The model under review builds one solid part; all positions refer to its coordinate system, in mm. A direction names the side the tool comes from. Give positions to 0.01 mm unless a question says otherwise; leave off trailing zeros. Order: outer loops, then holes, each group sorted by start corner. A loop starts at its lowest first (then second) coordinate and runs counter-clockwise, first axis right, second up. Notation, with made-up numbers: (43.25, 17) - (87.25, 17) arc R14 ccw to (87.25, 32) - close; hole circle Ø2 at (19, 38.25). An arc over 180 degrees is marked (long way). Put each result on its own line as item: value.
Autodesk Inventor part; units mm, degrees
ref_plane "YZ Plane" through (0, 0, 0) normal (1, 0, 0) x (0, 1, 0)
ref_plane "XZ Plane" through (0, 0, 0) normal (0, 1, 0) x (-1, 0, 0)
ref_plane "XY Plane" through (0, 0, 0) normal (0, 0, 1) x (1, 0, 0)
ref_plane "Arbeitsebene1" through (0, 0, 0) normal (0, 0, 1) x (1, 0, 0)
sketch "Skizze1" plane through (0, 0, 0) normal (0, 0, 1) x (1, 0, 0)
  line L0 (31.9586, -24.4) -> (31.9586, -21.8494)
  line L1 (31.9586, -24.4) -> (35.5793, -24.4)
  arc A0 (35.5793, -24.4) -> (36.5793, -23.4) centre (35.5793, -23.4) ccw
  line L2 (36.5793, -23.4) -> (36.5793, 14.6)
  arc A1 (36.5793, 14.6) -> (35.5793, 15.6) centre (35.5793, 14.6) ccw
  line L3 (35.5793, 15.6) -> (31.5586, 15.6)
  line L4 (31.5586, 15.6) -> (31.5586, -0.3724)
  arc A2 (32.766, -2.6793) -> (31.5586, -0.3724) centre (29.9586, -2.6793) ccw
  line L5 (32.766, -2.6793) -> (32.766, -19.8793)
  arc A3 (31.9586, -21.8494) -> (32.766, -19.8793) centre (29.9586, -19.8793) ccw
  line L6 (20.9586, -22.6867) -> (20.9586, -24.4)
  line L7 (20.9586, -22.6867) -> (16.1586, -22.6867)
  arc A4 (13.3512, -19.8793) -> (16.1586, -22.6867) centre (16.1586, -19.8793) ccw
  line L8 (13.3512, -19.8793) -> (13.3512, -2.6793)
  arc A5 (14.5586, -0.3724) -> (13.3512, -2.6793) centre (16.1586, -2.6793) ccw
  line L9 (14.5586, -0.3724) -> (14.5586, 15.6)
  line L10 (14.5586, 15.6) -> (10.5793, 15.6)
  arc A6 (10.5793, 15.6) -> (9.5793, 14.6) centre (10.5793, 14.6) ccw
  line L11 (9.5793, 14.6) -> (9.5793, -23.4)
  arc A7 (9.5793, -23.4) -> (10.5793, -24.4) centre (10.5793, -23.4) ccw
  line L12 (10.5793, -24.4) -> (20.9586, -24.4)
  circle A8 centre (12.0668, 4.4966) radius 1.4
  line L13 (31.5586, 15.6) -> (14.5586, 15.6)
  line L14 (31.9586, -24.4) -> (20.9586, -24.4)
  line L15 (10.5793, 15.6) -> (9.5793, 15.6)
  line L16 (9.5793, 15.6) -> (9.5793, 14.6)
  line L17 (35.5793, 15.6) -> (36.5793, 15.6)
  line L18 (36.5793, 15.6) -> (36.5793, 14.6)
  line L19 (9.5793, -23.4) -> (9.5793, -24.4)
  line L20 (9.5793, -24.4) -> (10.5793, -24.4)
  line L21 (35.5793, -24.4) -> (36.5793, -24.4)
  line L22 (36.5793, -24.4) -> (36.5793, -23.4)
extrude "Extrusion1" add sketch "Skizze1" along normal blind 2 contours L14 L6 L7 A4 L8 A5 L9 L13 L4 A2 L5 A3 L0 | L0 A3 L5 A2 L4 L3 A1 L2 A0 L1 | A0 L22 L21 | L12 A7 L11 A6 L10 L9 A5 L8 A4 L7 L6 | L20 L19 A7 | A1 L17 L18 | L16 L15 A6 | A8
ref_plane "Arbeitsebene2" through (0, 0, 0) normal (0, 0, 1) x (1, 0, 0)
sketch "Skizze2" plane through (0, 0, 2) normal (0, 0, 1) x (1, 0, 0)
  arc A0 (35.5793, -24.4) -> (36.5793, -23.4) centre (35.5793, -23.4) ccw
  line L0 (36.5793, -23.4) -> (36.5793, 14.6)
  arc A1 (36.5793, 14.6) -> (35.5793, 15.6) centre (35.5793, 14.6) ccw
  line L1 (35.5793, 15.6) -> (10.5793, 15.6)
  arc A2 (10.5793, 15.6) -> (9.5793, 14.6) centre (10.5793, 14.6) ccw
  line L2 (9.5793, 14.6) -> (9.5793, -23.4)
  arc A3 (9.5793, -23.4) -> (10.5793, -24.4) centre (10.5793, -23.4) ccw
  line L3 (10.5793, -24.4) -> (35.5793, -24.4)
  line L4 (34.0793, 13.1) -> (34.0793, -21.9)
  line L5 (34.0793, -21.9) -> (12.0793, -21.9)
  line L6 (12.0793, -21.9) -> (12.0793, 13.1)
  line L7 (12.0793, 13.1) -> (34.0793, 13.1)
  point P0 (8.0712, 15)
  point P1 (8.0712, -15)
  point P2 (38.0712, 15)
  point P3 (38.0712, -15)
  dimension "d21" = 2.5
hole "Bohrung1" at (34.0793, 13.1, 2) at (34.0793, -21.9, 2) at (12.0793, -21.9, 2) at (12.0793, 13.1, 2) direction (0, 0, -1) diameter 3.2 end through all
sketch "Skizze4" plane through (0, 0, 0) normal (0, 0, -1) x (-1, 0, 0)
  circle A0 centre (-34.0793, 13.1) radius 1.4
  circle A1 centre (-34.0793, -21.9) radius 1.4
  line L0 (-31.9586, -24.4) -> (-31.9586, -21.8494)
  line L1 (-31.9586, -24.4) -> (-35.5793, -24.4)
  arc A2 (-36.5793, -23.4) -> (-35.5793, -24.4) centre (-35.5793, -23.4) ccw
  line L2 (-36.5793, -23.4) -> (-36.5793, 14.6)
  arc A3 (-35.5793, 15.6) -> (-36.5793, 14.6) centre (-35.5793, 14.6) ccw
  line L3 (-35.5793, 15.6) -> (-31.5586, 15.6)
  line L4 (-31.5586, 15.6) -> (-31.5586, -0.3724)
  arc A4 (-31.5586, -0.3724) -> (-32.766, -2.6793) centre (-29.9586, -2.6793) ccw
  line L5 (-32.766, -2.6793) -> (-32.766, -19.8793)
  arc A5 (-32.766, -19.8793) -> (-31.9586, -21.8494) centre (-29.9586, -19.8793) ccw
  circle A6 centre (-12.0793, -21.9) radius 1.4
  circle A7 centre (-12.0793, 13.1) radius 1.4
  line L6 (-20.9586, -22.6867) -> (-20.9586, -24.4)
  line L7 (-20.9586, -22.6867) -> (-16.1586, -22.6867)
  arc A8 (-16.1586, -22.6867) -> (-13.3512, -19.8793) centre (-16.1586, -19.8793) ccw
  line L8 (-13.3512, -19.8793) -> (-13.3512, -2.6793)
  arc A9 (-13.3512, -2.6793) -> (-14.5586, -0.3724) centre (-16.1586, -2.6793) ccw
  line L9 (-14.5586, -0.3724) -> (-14.5586, 15.6)
  line L10 (-14.5586, 15.6) -> (-10.5793, 15.6)
  arc A10 (-9.5793, 14.6) -> (-10.5793, 15.6) centre (-10.5793, 14.6) ccw
  line L11 (-9.5793, 14.6) -> (-9.5793, -23.4)
  arc A11 (-10.5793, -24.4) -> (-9.5793, -23.4) centre (-10.5793, -23.4) ccw
  line L12 (-10.5793, -24.4) -> (-20.9586, -24.4)
  circle A12 centre (-12.0668, 4.4966) radius 1.4
  line L13 (-31.0586, -0.651) -> (-31.0586, 16.1)
  line L14 (-31.0586, 16.1) -> (-35.5793, 16.1)
  arc A13 (-35.5793, 16.1) -> (-37.0793, 14.6) centre (-35.5793, 14.6) ccw
  line L15 (-37.0793, 14.6) -> (-37.0793, -23.4)
  arc A14 (-37.0793, -23.4) -> (-35.5793, -24.9) centre (-35.5793, -23.4) ccw
  line L16 (-35.5793, -24.9) -> (-31.4586, -24.9)
  line L17 (-31.4586, -24.9) -> (-31.4586, -21.6326)
  arc A15 (-32.266, -19.8793) -> (-31.4586, -21.6326) centre (-29.9586, -19.8793) ccw
  line L18 (-32.266, -19.8793) -> (-32.266, -2.6793)
  arc A16 (-31.0586, -0.651) -> (-32.266, -2.6793) centre (-29.9586, -2.6793) ccw
  line L19 (-15.0586, 16.1) -> (-15.0586, -0.651)
  arc A17 (-13.8512, -2.6793) -> (-15.0586, -0.651) centre (-16.1586, -2.6793) ccw
  line L20 (-13.8512, -2.6793) -> (-13.8512, -19.8793)
  arc A18 (-16.1586, -22.1867) -> (-13.8512, -19.8793) centre (-16.1586, -19.8793) ccw
  line L21 (-16.1586, -22.1867) -> (-21.4586, -22.1867)
  line L22 (-21.4586, -24.4607) -> (-21.4586, -24.9)
  line L23 (-21.4586, -24.9) -> (-10.5793, -24.9)
  arc A19 (-10.5793, -24.9) -> (-9.0793, -23.4) centre (-10.5793, -23.4) ccw
  line L24 (-9.0793, -23.4) -> (-9.0793, 14.6)
  arc A20 (-9.0793, 14.6) -> (-10.5793, 16.1) centre (-10.5793, 14.6) ccw
  line L25 (-10.5793, 16.1) -> (-15.0586, 16.1)
  line L26 (-31.0586, 15.6607) -> (-15.0586, 15.6607)
  line L27 (-31.4586, -24.4607) -> (-21.4586, -24.4607)
  line L28 (-15.0586, -0.651) -> (-31.0586, -0.651)
  line L29 (-20.9586, -22.6867) -> (-20.9586, -22.1867)
  line L30 (-20.9586, -22.1867) -> (-31.9586, -22.1867)
  point P0 (0, 0)
  point P1 (-31.4586, -22.1867)
  dimension "d22" = 0.5
  dimension "d23" = 0.5
extrude "Extrusion2" add sketch "Skizze4" along normal blind 3 contours L17 A15 L18 A16 L28 A17 L20 A18 L21 L30
fillet "Rundung2" radius 4 4 edges at (9.5793, 15.6, 1) (36.5793, 15.6, 1) (9.5793, -24.4, 1) (36.5793, -24.4, 1)
sketch "Skizze5" plane through (0, 0, 0) normal (0, 0, -1) x (-1, 0, 0)
  circle A0 centre (-23.0793, -4.4) radius 4.25
  circle A1 centre (-12.0668, 4.4966) radius 1.4
  circle A2 centre (-34.0668, 4.4966) radius 1.4
  circle A3 centre (-12.0793, 13.1) radius 1.4
  circle A4 centre (-34.0793, -21.9) radius 1.4
  circle A5 centre (-34.0793, 13.1) radius 1.4
  circle A6 centre (-12.0793, -21.9) radius 1.4
  arc A7 (-29.0793, 13.6) -> (-31.0793, 15.6) centre (-31.0793, 13.6) ccw
  line L0 (-32.5793, 15.6) -> (-31.0793, 15.6)
  arc A8 (-32.5793, 15.6) -> (-36.5793, 11.6) centre (-32.5793, 11.6) ccw
  line L1 (-36.5793, -20.4) -> (-36.5793, 11.6)
  arc A9 (-36.5793, -20.4) -> (-32.5793, -24.4) centre (-32.5793, -20.4) ccw
  line L2 (-13.5793, -24.4) -> (-32.5793, -24.4)
  arc A10 (-13.5793, -24.4) -> (-9.5793, -20.4) centre (-13.5793, -20.4) ccw
  line L3 (-9.5793, 11.6) -> (-9.5793, -20.4)
  arc A11 (-9.5793, 11.6) -> (-13.5793, 15.6) centre (-13.5793, 11.6) ccw
  line L4 (-15.0793, 15.6) -> (-13.5793, 15.6)
  arc A12 (-15.0793, 15.6) -> (-17.0793, 13.6) centre (-15.0793, 13.6) ccw
  line L5 (-17.0793, 13.6) -> (-17.0793, 5.6)
  arc A13 (-19.0793, 3.6) -> (-17.0793, 5.6) centre (-19.0793, 5.6) ccw
  line L6 (-19.0793, 3.6) -> (-27.0793, 3.6)
  arc A14 (-29.0793, 5.6) -> (-27.0793, 3.6) centre (-27.0793, 5.6) ccw
  line L7 (-29.0793, 5.6) -> (-29.0793, 13.6)
  line L8 (-32.5793, 15.6) -> (-13.5793, 15.6)
  point P0 (0, 0)
extrude "Extrusion3" cut sketch "Skizze5" against normal blind 10 contours A7 L8 A12 L5 A13 L6 A14 L7
properties part number "00_ESP32_XIAO_Adapter_lid"
(1) Clearance check with flat-ended pins moving along their axes: pin 1 Ø2.5 at (x, z) = (23, -1) entering from +Y; pin 2 Ø1 at (x, z) = (31.5, -1.5) entering from -Y; pin 3 Ø0.9 at (y, z) = (-11.5, -1.5) entering from -X; pin 4 Ø5 at (x, y) = (34.08, 13.1) entering from +Z. State where each tip first meets the part, or that it passes through.
The answers:
pin 1: y = 3.6
pin 2: y = -22.19
pin 3: x = 13.85
pin 4: z = 2
(2) Take a section at B-B, the plane z = -2.3. Write out the cut boundary in (x, y), then the cut area to 3 significant figures.
The answers:
outline: (13.85, -19.88) arc R2.31 ccw to (16.16, -22.19) - (31.46, -22.19) - (31.46, -21.63) arc R2.31 ccw to (32.27, -19.88) - (32.27, -2.68) arc R2.31 ccw to (31.06, -0.65) - (15.06, -0.65) arc R2.31 ccw to (13.85, -2.68) - close
area: 393 mm^2
(3) Wall thickness on L1, parallel to X at y = 12, z = 1.05; L2, parallel to X at y = 13.1, z = 1.2; L3, parallel to Y at x = 11.5, z = 0.7: over which ranges is each line inside the solid? List them lowest first.
The answers:
L1: 9.6 to 10.92, 13.24 to 17.08, 29.08 to 32.92, 35.24 to 36.56
L2: 9.87 to 10.48, 13.68 to 17.08, 29.08 to 32.48, 35.68 to 36.29
L3: -23.82 to -23.39, -20.41 to 11.61, 14.59 to 15.02
(4) Take a section at C-C, the plane x = 22.25. Write out the cut boundary in (y, z).
The answers:
outline: (-24.4, 0) - (-22.19, 0) - (-22.19, -3) - (-0.65, -3) - (-0.65, 0) - (3.6, 0) - (3.6, 2) - (-24.4, 2) - close
(5) The part is to be moulded in two halves that separate along Y. For faces 1 (the cylindrical face through (11.599, 11.574, 0.986)), 2 (the flat face through (24, -22.187, -1)), 3 (the cylindrical face through (33.599, -23.426, 0.986)), 4 (the cylindrical face through (17.68, 4.17, 0.99)), say which applies: pulls with the +Y half, pulls with the -Y half, needs draft (parallel to the pull), parting line crosses it, or undercut.
The answers:
face 1: undercut
face 2: pulls with the -Y half
face 3: undercut
face 4: pulls with the +Y half
(6) For faces 5 (the cylindrical face through (32.049, -20.857, -1.479)), 6 (the cylindrical face through (14.185, -1.484, -1.479)), 7 (the cylindrical face through (14.509, -21.493, -1.479)), 8 (the flat face through (32.266, -11, -1)), 9 (the cylindrical face through (28.51, 4.2, 0.99)), list the 3-axis set-ups (+Z, -Z, +X, -X, +Y, -Y) from which the entire face can be reached by the end or side of a thin tool; tool diameter is ignored.
The answers:
face 5: -Z, +X, -Y
face 6: -Z, -X, +Y
face 7: -Z, -X, -Y
face 8: -Z, +X, +Y, -Y
face 9: +Z, -Z, +Y
(7) Take a section at A-A, the plane y = 9.5. Write out the cut boundary in (x, z).
The answers:
outline: (9.58, 0) - (17.08, 0) - (17.08, 2) - (9.58, 2) - close; (29.08, 0) - (36.58, 0) - (36.58, 2) - (29.08, 2) - close
(8) Take a section at D-D, the plane x = 33.25. Write out the cut boundary in (y, z).
The answers:
outline: (-24.34, 0) - (-23.27, 0) - (-23.27, 2) - (-24.34, 2) - close; (-20.53, 0) - (11.73, 0) - (11.73, 2) - (-20.53, 2) - close; (14.47, 0) - (15.54, 0) - (15.54, 2) - (14.47, 2) - close
